Autodesk Inventor part; units mm, degrees
ref_plane "YZ Plane" through (0, 0, 0) normal (1, 0, 0) x (0, 1, 0)
ref_plane "XZ Plane" through (0, 0, 0) normal (0, 1, 0) x (-1, 0, 0)
ref_plane "XY Plane" through (0, 0, 0) normal (0, 0, 1) x (1, 0, 0)
sketch "Sketch1" plane through (0, 0, 0) normal (0, 1, 0) x (-1, 0, 0)
  line L0 (0, 0) -> (15.875, 0)
  line L1 (15.875, 0) -> (15.875, -38.1)
  line L2 (15.875, -38.1) -> (0, -38.1)
  line L3 (0, -38.1) -> (0, 0)
  line L4 (0, -19.05) -> (7.6962, -19.05) construction
  line L5 (7.6962, -19.05) -> (12.4714, -19.05) construction
  line L6 (12.4714, -19.05) -> (12.4714, -31.75) construction
  circle A0 centre (12.4714, -31.75) radius 1.5875
  line L7 (7.6962, -19.05) -> (7.0104, -19.05) construction
  line L8 (7.0104, -19.05) -> (7.0104, -23.8125) construction
  circle A1 centre (7.0104, -23.8125) radius 0.8001
  circle A2 centre (12.4714, -6.35) radius 1.5875
  circle A3 centre (7.0104, -14.2875) radius 0.8001
  dimension "d0" = 15.875
  dimension "d1" = 38.1
  dimension "d2" = 7.6962
  dimension "d3" = 4.7752
  dimension "d4" = 12.7
  dimension "d5" = 3.175
  dimension "d7" = 4.7625
  dimension "d8" = 1.6002
  dimension "d11" = 7.0104
extrude "Extrusion1" add sketch "Sketch1" along normal blind 6.35
properties part number "limitSwitchMount"
Geometry check sheet. Reference: the model listing, model coordinates, mm. Round coordinates to 2 decimals unless told otherwise and drop trailing zeros. Order: outer loops, then holes, each group sorted by start corner. A loop starts at its lowest first (then second) coordinate and runs counter-clockwise, first axis right, second up. Notation, with made-up numbers: M -39,66 L -34,66 A10 ccw -34,77 Z; hole C 34.5,39 d8. An arc over 180 degrees is marked long. Answer in a Markdown table with one row per item.
(1) Draft check along Z on faces 1 (the face through (-8, 3, 0)), 2 (the face through (0, 3, -19)), 3 (the face through (-13.32, 3.13, -33.09)), 4 (the face through (-13.938, 3.131, -5.742)). Enter one of: released by +Z, released by -Z, zero draft, split by the parting line, or undercut.
Responses:
| item | result |
|---|---|
| face 1 | released by +Z |
| face 2 | zero draft |
| face 3 | undercut |
| face 4 | undercut |
(2) Sectioned sample at C-C, the plane z = -30.5. Record the cut outline in (x, y) (3 decimals), and give its area (3 significant figures).
Responses:
| item | result |
|---|---|
| outline | M -15.875,0 L -13.45,0 L -13.45,6.35 L -15.875,6.35 Z; M -11.493,0 L 0,0 L 0,6.35 L -11.493,6.35 Z |
| area | 88.4 mm² |
(3) Scan lines: probe 1 along Z at (x, y) = (-12.5, 1.75); probe 2 along Z at (x, y) = (-7, 3.25); probe 3 along X at (y, z) = (5.5, -6) (3 decimals). Record each from-to range of solid material in increasing order. Write a range as from..to.
Responses:
| item | result |
|---|---|
| probe 1 | z = -38.1..-33.34, -30.16..-7.94, -4.76..0 |
| probe 2 | z = -38.1..-24.61, -23.01..-15.09, -13.49..0 |
| probe 3 | x = -15.875..-14.02, -10.923..0 |
(4) Sectioned sample at B-B, the plane y = 6. State how many separate pieces and enclosed holes the cut face has, and give its area (3 significant figures).
Responses:
| item | result |
|---|---|
| separate pieces | 1 |
| enclosed holes | 4 |
| area | 585 mm² |
(5) Go/stop test with a flat-tipped pin: P1, Ø4, axis at x = -12.47, z = -6.35, coming from the -Y side. Record where the tip stops, or that it passes through.
Responses:
| item | result |
|---|---|
| P1 | stops at y = 0 |
(6) Sectioned sample at A-A, the plane z = -6.35. Record the cut outline in (x, y) (3 decimals), and give its area (3 significant figures).
Responses:
| item | result |
|---|---|
| outline | M -15.875,0 L -14.059,0 L -14.059,6.35 L -15.875,6.35 Z; M -10.884,0 L 0,0 L 0,6.35 L -10.884,6.35 Z |
| area | 80.6 mm² |
